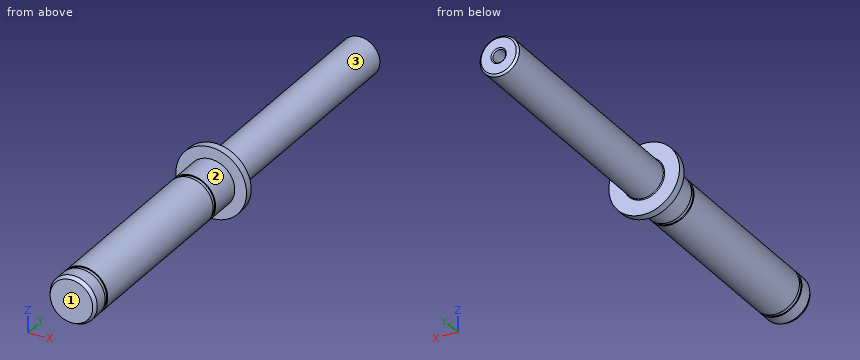
from build123d import *

# Parameters (mm, degrees)
ZKOSEN_1_SIZE   = 0.5
ZKOSEN_2_SIZE   = 1
ZKOSEN_2_SIZE2  = 0.577350269
ZAOBLIT3_R      = 0.2
M4_Z_VIT1_D     = 3.3
M4_Z_VIT1_DEPTH = 12
M4_Z_VIT1_TIP   = 0.991420021
ZKOSEN_4_SIZE   = 0.3


with BuildPart() as part:
    # Skica1 → Rotovat1 (revolve)
    with BuildSketch(Plane.XY, mode=Mode.PRIVATE) as rotovat1_sk:
        Polygon((-6, 0), (-6, 4.4), (-5.75, 4.4), (-5.75, 5.5), (-6, 5.5), (-6, 51.1), (-5.75, 51.1), (-5.75, 52.2), (-6, 52.2), (-6, 60.5), (-9, 60.5), (-9, 62.5), (-5, 62.5), (-5, 125.5), (0, 125.5), (0, 0), align=None)
    revolve(rotovat1_sk.sketch.rotate(Axis((0, 0, 0), (0, 1, 0)), 270), axis=Axis((0, 0, 0), (0, 1, 0)))

    # Zkosení1
    zkosen_1_edges = [part.edges().sort_by_distance(p)[0] for p in [
        (0, 125.5, 5),
    ]]
    chamfer(zkosen_1_edges, length=ZKOSEN_1_SIZE)

    # Zkosení2
    zkosen_2_edges = [part.edges().sort_by_distance(p)[0] for p in [
        (0, 0, 6),
    ]]
    zkosen_2_side = [part.faces().sort_by_distance(p)[0] for p in [
        (0, 2.2, 6),
    ]]
    chamfer(zkosen_2_edges, length=ZKOSEN_2_SIZE, length2=ZKOSEN_2_SIZE2, reference=zkosen_2_side[0])

    # Zaoblit3
    zaoblit3_edges = [part.edges().sort_by_distance(p)[0] for p in [
        (0, 62.5, 5),
    ]]
    fillet(zaoblit3_edges, radius=ZAOBLIT3_R)

    # M4 závit1
    with Locations(Plane(origin=(0, 125.5, 0), x_dir=(1, 0, 0), z_dir=(0, 1, 0))):
        with Locations((0, 0)):
            Hole(M4_Z_VIT1_D / 2, depth=M4_Z_VIT1_DEPTH)
            with Locations((0, 0, -(M4_Z_VIT1_DEPTH + M4_Z_VIT1_TIP / 2))):  # 118° drill point
                Cone(0, M4_Z_VIT1_D / 2, M4_Z_VIT1_TIP, mode=Mode.SUBTRACT)

    # Zkosení4
    zkosen_4_edges = [part.edges().sort_by_distance(p)[0] for p in [
        (1.65, 125.5, 0),
    ]]
    chamfer(zkosen_4_edges, length=ZKOSEN_4_SIZE)


solid = part.part
Model file for the job. Use its own axes, mm. Face numbers are marked on the shaded views. A direction names the side the tool comes from. Give positions to 0.01 mm unless a question says otherwise; leave off trailing zeros. Order: outer loops, then holes, each group sorted by start corner. A loop starts at its lowest first (then second) coordinate and runs counter-clockwise, first axis right, second up. Notation, with made-up numbers: (-15.75, 37) - (13.25, 37) arc R25 cw to (13.25, 73) - close; hole circle Ø7 at (59, 76). An arc over 180 degrees is marked (long way). Return JSON: item names as keys, results as strings.
1) Cut at B-B, the plane y = 13.5. Give the cut face in (x, z), plus the area to 3 significant figures.
Geometry says:
{"outline": "circle Ø12 at (0, 0)", "area": "113 mm²"}
2) Probe line 1 (Y direction, x = -5.5, z = 5); line 2 (X direction, y = 40, z = -1.75); line 3 (X direction, y = 123, z = 0). List the from-to ranges inside material, lowest first. Write a range as from..to.
Geometry says:
{"line 1": "60.5..62.5", "line 2": "-5.74..5.74", "line 3": "-5..-1.65, 1.65..5"}
3) Cut at A-A, the plane y = 97.5. Give the cut face in (x, z).
Geometry says:
{"outline": "circle Ø10 at (0, 0)"}
4) Flat gauge pins, fed straight in: P1, Ø3, axis at y = 81.5, z = 0, coming from the -X side; P2, Ø1, axis at y = 16.5, z = 1.5, coming from the +X side; P3, Ø3.5, axis at x = 1, z = -1.5, coming from the +Y side; P4, Ø1, axis at x = 5.5, z = -3, coming from the +Y side. Where does each tip first touch, or does it go through?
Geometry says:
{"P1": "x = -5", "P2": "x = 5.92", "P3": "y = 125.5", "P4": "y = 62.5"}
5) 3-axis set-ups, long thin cutter, end or side, ignore diameter. For the marked faces 1, 2 and 3: which of +Z, -Z, +X, -X, +Y, -Y reach the whole face in a straight line?
Geometry says:
{"face 1": "+Z, -Z, +X, -X, -Y", "face 2": "-Y", "face 3": "+Y"}
